Geometry check sheet. Reference: drawing and pictorial views, mm from the part's lowest x, y, z. A direction names the side the tool comes from. Coordinates: 2 decimals unless noted, no trailing zeros. Write each loop counter-clockwise with the first axis right and the second up, starting at its lowest first coordinate (ties: lowest second). Pieces come first, ordered by that corner, then holes. Notation, with made-up numbers: (-24, 9.25) - (27, 9.25) arc R27 ccw to (27, 32.25) - close; hole circle Ø2 at (84, -17.5). An arc over 180 degrees is marked (long way). Use one line per item in the form item = value. Start each with the question number.
(1) Tool access check on the marked faces 5 and 6. Record the directions out of +Z, -Z, +X, -X, +Y, -Y that give a thin tool (end or side, any length) a straight path to the whole face; none if there is none.
(2) Mould release check, pull along Y, two halves, no side actions. Record for the marked faces 1, 2, 3 and 4: released by +Y, released by -Y, zero draft, split by the parting line, or undercut.
(3) Material ranges on line 1 (Y direction, x = 43.5, z = 8.25); line 2 (X direction, y = 3, z = 8); line 3 (X direction, y = 7.5, z = 7.5) (1 decimal), recorded low to high. Write a range as [from, to].
(4) Gauge pin test, flat ends, axial feed: pin 1 Ø1.6 at (y, z) = (6, 4) entering from +X; pin 2 Ø2 at (x, y) = (51.5, 5.5) entering from +Z; pin 3 Ø1.5 at (y, z) = (1.5, 7.5) entering from +X (1 decimal); pin 4 Ø4 at (y, z) = (9.5, 3.5) entering from +X. Record the tip position at first contact, or that the pin passes through.
(5) Sectioned sample at A-A (z = 8.75). Count the separate pieces of the cut face and the enclosed holes in it, and give its area (3 significant figures).
(6) Sectioned sample at B-B (x = 18.5). Record the cut outline in (y, z).
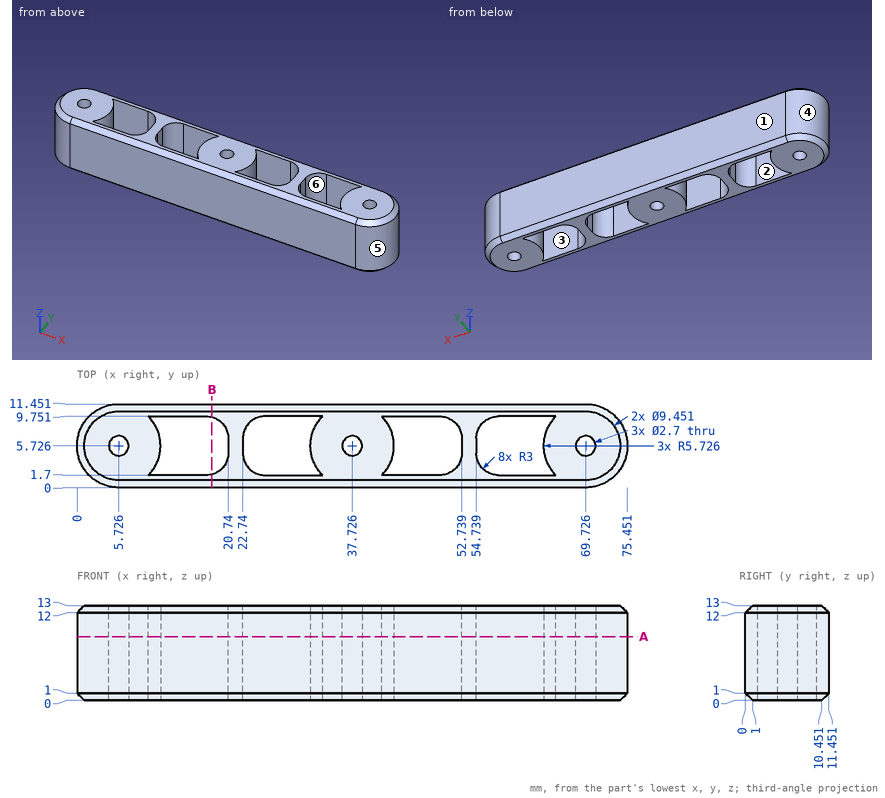
Answers below:
q1.face_5 = +Z, -Z, +X
q1.face_6 = +Z, -Z
q2.face_1 = released by +Y
q2.face_2 = undercut
q2.face_3 = undercut
q2.face_4 = split by the parting line
q3.line_1 = [0, 1.7], [9.75, 11.45]
q3.line_2 = [0.69, 10.76], [20.21, 23.27], [32.69, 42.76], [52.21, 55.27], [64.69, 74.76]
q3.line_3 = [0.3, 11.2], [20.6, 22.8], [32.3, 43.2], [52.6, 54.8], [64.3, 75.2]
q4.pin_1 = 75.45
q4.pin_2 = through
q4.pin_3 = 74.3
q4.pin_4 = 75.17
q5.separate_pieces = 1
q5.enclosed_holes = 7
q5.area = 519 mm2
q6.outline = (0, 1) - (1, 0) - (1.8, 0) - (1.8, 13) - (1, 13) - (0, 12) - close; (9.65, 0) - (10.45, 0) - (11.45, 1) - (11.45, 12) - (10.45, 13) - (9.65, 13) - close
